```python
from build123d import *

# Parameters (mm, degrees)
SKETCH1_W                                     = 98
SKETCH1_H                                     = 98
BOSS_EXTRUDE1_DEPTH                           = 3.175
SKETCH2_W                                     = 7.5
SKETCH2_H                                     = 7.5
CUT_EXTRUDE1_DEPTH                            = 70.369161917
F_4_CLEARANCE_HOLE1_D                         = 2.9464
M2_CLEARANCE_HOLE1_D                          = 2.2
CSK_FOR_4_FLAT_HEAD_MACHINE_SCREW1_AT_2_COUNT = 2
CSK_FOR_4_FLAT_HEAD_MACHINE_SCREW1_AT_2_PITCH = 74.5
CSK_FOR_4_FLAT_HEAD_MACHINE_SCREW1_AT_3_COUNT = 2
CSK_FOR_4_FLAT_HEAD_MACHINE_SCREW1_AT_3_PITCH = 105.358910397
CSK_FOR_4_FLAT_HEAD_MACHINE_SCREW1_AT_4_COUNT = 2
CSK_FOR_4_FLAT_HEAD_MACHINE_SCREW1_AT_4_PITCH = 74.5
CUT_EXTRUDE2_DEPTH                            = 70.369161917
SKETCH12_R                                    = 2.25
CUT_EXTRUDE3_DEPTH                            = 1.675
FILLET1_R                                     = 0.5


with BuildPart() as part:
    # Sketch1 → Boss-Extrude1 (new body)
    with BuildSketch(Plane(origin=(0, 0, 0), x_dir=(1, 0, 0), z_dir=(0, 1, 0))):
        Rectangle(SKETCH1_W, SKETCH1_H)
    extrude(amount=BOSS_EXTRUDE1_DEPTH)

    # Sketch2 → Cut-Extrude1 (cut, through all)
    with BuildSketch(Plane(origin=(0, 3.175, 0), x_dir=(1, 0, 0), z_dir=(0, 1, 0))):
        with Locations((45.25, 45.25)):
            Rectangle(SKETCH2_W, SKETCH2_H)
        with Locations((-45.25, 45.25)):
            Rectangle(SKETCH2_W, SKETCH2_H)
        with Locations((45.25, -45.25)):
            Rectangle(SKETCH2_W, SKETCH2_H)
        with Locations((-45.25, -45.25)):
            Rectangle(SKETCH2_W, SKETCH2_H)
    extrude(amount=-CUT_EXTRUDE1_DEPTH, mode=Mode.SUBTRACT)

    # #4 Clearance Hole1 (through all)
    with Locations(Plane(origin=(0, 3.175, 0), x_dir=(1, 0, 0), z_dir=(0, 1, 0))):
        with Locations((0, 0)):
            Hole(F_4_CLEARANCE_HOLE1_D / 2)

    # M2 Clearance Hole1 (through all)
    with Locations(Plane(origin=(0, 3.175, 0), x_dir=(1, 0, 0), z_dir=(0, 1, 0))):
        with Locations((-28.095, 35.095), (12.545, 35.095), (12.545, 8.425), (-28.095, 8.425)):
            Hole(M2_CLEARANCE_HOLE1_D / 2)

    # Sketch9 → CSK for #4 Flat Head Machine Screw1 (revolve, cut)
    with BuildSketch(Plane(origin=(37.25, 3.175, 37.25), x_dir=(0, 0, 1), z_dir=(1, 0, 0))):
        Polygon((0, 0), (0, 3.175), (1.63195, 3.175), (1.63195, 1.409834001), (2.8575, 0), align=None)
    csk_for_4_flat_head_machine_screw1 = revolve(axis=Axis((37.25, 9.525, 37.25), (0, -1, 0)), mode=Mode.SUBTRACT)

    # CSK for #4 Flat Head Machine Screw1 at 2: CSK for #4 Flat Head Machine Screw1 ×2
    with Locations(*[(-i * CSK_FOR_4_FLAT_HEAD_MACHINE_SCREW1_AT_2_PITCH, 0, 0) for i in range(1, CSK_FOR_4_FLAT_HEAD_MACHINE_SCREW1_AT_2_COUNT)]):
        add(csk_for_4_flat_head_machine_screw1, mode=Mode.SUBTRACT)

    # CSK for #4 Flat Head Machine Screw1 at 3: CSK for #4 Flat Head Machine Screw1 ×2
    with Locations(*[Vector(-0.7071067811865502, 0, -0.7071067811865448) * (i * CSK_FOR_4_FLAT_HEAD_MACHINE_SCREW1_AT_3_PITCH) for i in range(1, CSK_FOR_4_FLAT_HEAD_MACHINE_SCREW1_AT_3_COUNT)]):
        add(csk_for_4_flat_head_machine_screw1, mode=Mode.SUBTRACT)

    # CSK for #4 Flat Head Machine Screw1 at 4: CSK for #4 Flat Head Machine Screw1 ×2
    with Locations(*[(0, 0, -i * CSK_FOR_4_FLAT_HEAD_MACHINE_SCREW1_AT_4_PITCH) for i in range(1, CSK_FOR_4_FLAT_HEAD_MACHINE_SCREW1_AT_4_COUNT)]):
        add(csk_for_4_flat_head_machine_screw1, mode=Mode.SUBTRACT)

    # Sketch11 → Cut-Extrude2 (cut, through all)
    with BuildSketch(Plane(origin=(0, 3.175, 0), x_dir=(1, 0, 0), z_dir=(0, 1, 0))):
        Polygon((-49, -41.246), (-41.246, -41.246), (-41.246, -49), (-41.5, -49), (-41.5, -41.5), (-49, -41.5), align=None)
        Polygon((41.246, -49), (41.246, -41.246), (49, -41.246), (49, -41.5), (41.5, -41.5), (41.5, -49), align=None)
        Polygon((49, 41.246), (41.246, 41.246), (41.246, 49), (41.5, 49), (41.5, 41.5), (49, 41.5), align=None)
        Polygon((-41.246, 49), (-41.246, 41.246), (-49, 41.246), (-49, 41.5), (-41.5, 41.5), (-41.5, 49), align=None)
    extrude(amount=-CUT_EXTRUDE2_DEPTH, mode=Mode.SUBTRACT)

    # Sketch12 → Cut-Extrude3 (cut)
    with BuildSketch(Plane(origin=(0, 3.175, 0), x_dir=(1, 0, 0), z_dir=(0, 1, 0))):
        with Locations(Location((-28.095, 35.095, 0), (0, 0, 270))):
            Circle(SKETCH12_R)
        with Locations(Location((12.545, 35.095, 0), (0, 0, 270))):
            Circle(SKETCH12_R)
        with Locations(Location((12.545, 8.425, 0), (0, 0, 270))):
            Circle(SKETCH12_R)
        with Locations(Location((-28.095, 8.425, 0), (0, 0, 270))):
            Circle(SKETCH12_R)
    extrude(amount=-CUT_EXTRUDE3_DEPTH, mode=Mode.SUBTRACT)

    # Fillet1
    fillet1_edges = [part.edges().sort_by_distance(p)[0] for p in [
        (-28.095, 1.5, -37.345),
        (12.545, 1.5, -37.345),
        (12.545, 1.5, -10.675),
        (-28.095, 1.5, -10.675),
    ]]
    fillet(fillet1_edges, radius=FILLET1_R)


solid = part.part
```
The listing builds one solid part. Answer for the finished solid, in the listing's coordinates (mm). A direction names the side the tool comes from. Round coordinates to 2 decimals unless told otherwise and drop trailing zeros. Loops run counter-clockwise (first coordinate to the right, second up) from the corner with the lowest first, then second, coordinate; pieces in that order, holes last.
Q1. Given pin 1 Ø1.6 at (y, z) = (1.5, 45.5) entering from +X; pin 2 Ø1.6 at (y, z) = (2, 44) entering from -X; pin 3 Ø3 at (x, z) = (-28, -35.5) entering from +Y, each flat-ended and moving along its own axis, determine where each tip first touches the part or whether it passes through.
Q2. Which of the six approach directions +Z, -Z, +X, -X, +Y, -Y give full straight-line access (tool end or side, diameter ignored) to faces 5 (the face through (-27, 1.5, -34)), 6 (the face through (-45, 2, 41.246)), 7 (the face through (45, 2, 41.246)), 8 (the face through (49, 2, 1)), 9 (the face through (-1.405, 1.565, -0.443))?
Q3. For a pull along X with two mould halves and no side action, classify faces 1 (the face through (-1, 2, 49)), 2 (the face through (12.688, 0.739, -36.186)), 3 (the face through (-30.291, 2.596, -35.583)), 4 (the face through (-49, 2, 1)) as released by +X, released by -X, zero draft, split by the parting line, or undercut.
Q4. Section D-D, the plane y = 2.6 is taken. Count the separate pieces of the cut face and the enclosed holes in it, then the cut area to 3 significant figures.
Q5. Section B-B, the plane x = -37.25 is taken. Determine the outline of the cut face in (y, z) (1 decimal), then the cut area to 3 significant figures.
Q6. Section A-A, the plane x = 0 is taken. Determine the outline of the cut face in (y, z) (3 decimals).
Q7. Find the intervals of material crossed by line 1 (X direction, y = 0.7, z = 37.25); line 2 (Z direction, x = 0, y = 0.5), in increasing order.
Q8. Section C-C, the plane z = 0 is taken. Determine the outline of the cut face in (x, y) (3 decimals), then the cut area to 3 significant figures.
Completed:
1. pin 1: stops at x = 41.25
1. pin 2: stops at x = -41.25
1. pin 3: stops at y = 1.53
2. face 5: +Y
2. face 6: +Z, -X, +Y, -Y
2. face 7: +Z, +X, +Y, -Y
2. face 8: +Z, -Z, +X, +Y, -Y
2. face 9: +Y, -Y
3. face 1: zero draft
3. face 2: undercut
3. face 3: undercut
3. face 4: released by -X
4. separate pieces: 1
4. enclosed holes: 9
4. area: 9,220 mm2
5. outline: (0, -49) - (3.2, -49) - (3.2, -40.1) - (1.8, -38.9) - (0, -38.9) - close; (0, -35.6) - (1.8, -35.6) - (3.2, -34.4) - (3.2, 34.4) - (1.8, 35.6) - (0, 35.6) - close; (0, 38.9) - (1.8, 38.9) - (3.2, 40.1) - (3.2, 49) - (0, 49) - close
5. area: 287 mm2
6. outline: (0, -49) - (3.175, -49) - (3.175, -1.473) - (0, -1.473) - close; (0, 1.473) - (3.175, 1.473) - (3.175, 49) - (0, 49) - close
7. line 1: x = -49 to -38.88, -35.62 to 35.62, 38.88 to 49
7. line 2: z = -49 to -1.47, 1.47 to 49
8. outline: (-49, 0) - (-1.473, 0) - (-1.473, 3.175) - (-49, 3.175) - close; (1.473, 0) - (49, 0) - (49, 3.175) - (1.473, 3.175) - close
8. area: 302 mm2
